Read the model definition and answer for the solid it produces. Units are mm, in the model's axes. A direction names the side the tool comes from. Coordinates: 2 decimals unless noted, no trailing zeros. Write each loop counter-clockwise with the first axis right and the second up, starting at its lowest first coordinate (ties: lowest second). Pieces come first, ordered by that corner, then holes. Notation, with made-up numbers: (-24, 10.25) -> (-12, 10.25) arc R31 ccw to (-12, 37.25) -> close; hole circle Ø2 at (24, 89). An arc over 180 degrees is marked (long way). Return JSON: item names as keys, results as strings.
from build123d import *

# Parameters (mm, degrees)
SKETCH_1_W           = 94
SKETCH_1_H           = 26
SKETCH_1_R           = 0.6
EXTRUDE_1_DEPTH      = 8
SKETCH_2_W           = 4.7
SKETCH_2_H           = 8.9
SKETCH_2_W_2         = 59.6
SKETCH_2_H_2         = 6.6
CUT_EXTRUDE_1_DEPTH  = 50.416596402
SKETCH_3_R           = 1.5
CUT_EXTRUDE_2_DEPTH  = 50.416596402
SKETCH_5_W           = 7.8
SKETCH_5_H           = 2.6
SKETCH_5_W_2         = 8.6
SKETCH_5_H_2         = 2
CUT_EXTRUDE_4_DEPTH  = 6
SKETCH_5_3_W         = 15.6
SKETCH_5_3_H         = 2
CUT_EXTRUDE_5_DEPTH  = 20
SKETCH_6_W           = 70
SKETCH_6_H           = 19.6
SKETCH_6_W_2         = 18.8
SKETCH_6_H_2         = 3
SKETCH_6_W_3         = 82.8
SKETCH_6_H_3         = 11
SKETCH_6_W_4         = 3.2
SKETCH_6_H_4         = 5.2
CUT_EXTRUDE_12_DEPTH = 2
SKETCH_7_W           = 6.7
SKETCH_7_H           = 7.7
CUT_EXTRUDE_13_DEPTH = 0.5
SKETCH_8_W           = 7.4
SKETCH_8_H           = 5.4
SKETCH_8_W_2         = 15.6
SKETCH_8_H_2         = 1.5
EXTRUDE_2_DEPTH      = 2.1
SKETCH_10_W          = 19.8
SKETCH_10_H          = 1.9
SKETCH_10_W_2        = 11.8
SKETCH_10_H_2        = 4.2
EXTRUDE_3_DEPTH      = 2
EXTRUDE_4_REACH      = 53.894
SKETCH_12_W          = 100
SKETCH_12_H          = 32.2
SKETCH_12_W_2        = 94
SKETCH_12_H_2        = 26.1
SKETCH_12_3_W        = 4.3
SKETCH_12_3_H        = 3
SKETCH_12_3_W_2      = 1
SKETCH_12_3_W_3      = 3.2
SKETCH_12_3_H_2      = 5.2
CUT_EXTRUDE_16_DEPTH = 54.133887492
SKETCH_13_W          = 94
SKETCH_13_H          = 0.1
EXTRUDE_5_DEPTH      = 8
SKETCH_14_W          = 1
SKETCH_14_H          = 8
CUT_EXTRUDE_17_DEPTH = 0.5
SKETCH_15_W          = 100
SKETCH_15_H          = 4
EXTRUDE_6_DEPTH      = 2
SKETCH_16_W          = 12
SKETCH_16_H          = 3.1
CUT_EXTRUDE_18_DEPTH = 55.479445665
SKETCH_17_R          = 1
CUT_EXTRUDE_19_DEPTH = 55.221859061
CUT_EXTRUDE_20_REACH = 104.313
SKETCH_18_W          = 8.9
SKETCH_18_H          = 4.7
SKETCH_19_W          = 4
SKETCH_19_H          = 1.5
CUT_EXTRUDE_21_DEPTH = 55.479445665


with BuildPart() as part:
    # 草图1 → 凸台-拉伸1 (new body)
    with BuildSketch(Plane(origin=(0, 0, 0), x_dir=(1, 0, 0), z_dir=(0, 1, 0))):
        Rectangle(SKETCH_1_W, SKETCH_1_H)
        with Locations(Location((-44, 10, 0), (0, 0, 270))):
            Circle(SKETCH_1_R, mode=Mode.SUBTRACT)
        with Locations(Location((-44, -10, 0), (0, 0, 270))):
            Circle(SKETCH_1_R, mode=Mode.SUBTRACT)
        with Locations(Location((44, 10, 0), (0, 0, 270))):
            Circle(SKETCH_1_R, mode=Mode.SUBTRACT)
        with Locations(Location((44, -10, 0), (0, 0, 270))):
            Circle(SKETCH_1_R, mode=Mode.SUBTRACT)
    extrude(amount=EXTRUDE_1_DEPTH)

    # 草图2 → 切除-拉伸1 (cut, through all)
    with BuildSketch(Plane.XZ):
        with Locations((-44.65, 2.65)):
            Rectangle(SKETCH_2_W, SKETCH_2_H)
        with Locations((-4.8, 0)):
            Rectangle(SKETCH_2_W_2, SKETCH_2_H_2)
    extrude(amount=-CUT_EXTRUDE_1_DEPTH, mode=Mode.SUBTRACT)

    # 草图3 → 切除-拉伸2 (cut, through all)
    with BuildSketch(Plane(origin=(0, 0, 0), x_dir=(-1, 0, 0), z_dir=(0, -1, 0))):
        with Locations(Location((27.5, -10, 0), (0, 0, 90))):
            Circle(SKETCH_3_R)
    extrude(amount=-CUT_EXTRUDE_2_DEPTH, mode=Mode.SUBTRACT)

    # 草图5 → 切除-拉伸4 (cut)
    with BuildSketch(Plane.XY.offset(13)):
        with Locations((-37.2, 6.7)):
            Rectangle(SKETCH_5_W, SKETCH_5_H)
        with Locations((-27.5, 7)):
            Rectangle(SKETCH_5_W_2, SKETCH_5_H_2)
    extrude(amount=-CUT_EXTRUDE_4_DEPTH, mode=Mode.SUBTRACT)

    # 草图5<3> → 切除-拉伸5 (cut)
    with BuildSketch(Plane.XY.offset(13)):
        with Locations((32.9, 7)):
            Rectangle(SKETCH_5_3_W, SKETCH_5_3_H)
    extrude(amount=-CUT_EXTRUDE_5_DEPTH, mode=Mode.SUBTRACT)

    # 草图6 → 切除-拉伸12 (cut)
    with BuildSketch(Plane(origin=(0, 8, 0), x_dir=(1, 0, 0), z_dir=(0, 1, 0))):
        with Locations((-7.8, 2.7)):
            Rectangle(SKETCH_6_W, SKETCH_6_H)
        with Locations((36.6, 0)):
            Rectangle(SKETCH_6_W_2, SKETCH_6_H_2)
        with Locations((0.3, -7)):
            Rectangle(SKETCH_6_W_3, SKETCH_6_H_3)
        with Locations((-44.4, 5.4)):
            Rectangle(SKETCH_6_W_4, SKETCH_6_H_4)
    extrude(amount=-CUT_EXTRUDE_12_DEPTH, mode=Mode.SUBTRACT)

    # 草图7 → 切除-拉伸13 (cut)
    with BuildSketch(Plane(origin=(0, 6, 0), x_dir=(1, 0, 0), z_dir=(0, 1, 0))):
        with Locations((-27.35, 7.15)):
            Rectangle(SKETCH_7_W, SKETCH_7_H)
    extrude(amount=-CUT_EXTRUDE_13_DEPTH, mode=Mode.SUBTRACT)

    # 草图8 → 凸台-拉伸2 (add)
    with BuildSketch(Plane.XY.offset(13)):
        with Locations((-37.2, 2.7)):
            Rectangle(SKETCH_8_W, SKETCH_8_H)
        with Locations((32.9, 0.75)):
            Rectangle(SKETCH_8_W_2, SKETCH_8_H_2)
    extrude(amount=EXTRUDE_2_DEPTH)

    # 草图10 → 凸台-拉伸3 (add)
    with BuildSketch(Plane.ZY.offset(47)):
        with Locations((0, 0.95)):
            Rectangle(SKETCH_10_W, SKETCH_10_H)
        with Locations((0, 2.1)):
            Rectangle(SKETCH_10_W_2, SKETCH_10_H_2)
    extrude(amount=EXTRUDE_3_DEPTH)

    # 凸台-拉伸4: up to this face of the body (flat: up to its plane)
    extrude_4_end = Plane(part.part.faces().sort_by_distance((-45.999719539, 0, 11.45))[0])
    # 草图12 → 凸台-拉伸4 (add, up to the picked face)
    with BuildSketch(Plane(origin=(0, 8, 0), x_dir=(1, 0, 0), z_dir=(0, 1, 0)), mode=Mode.PRIVATE) as extrude_4_sk1:
        Rectangle(SKETCH_12_W, SKETCH_12_H)
        with Locations((0, -0.05)):
            Rectangle(SKETCH_12_W_2, SKETCH_12_H_2, mode=Mode.SUBTRACT)
    extrude_4_tool1 = split(extrude(extrude_4_sk1.sketch, amount=-EXTRUDE_4_REACH, mode=Mode.PRIVATE), bisect_by=extrude_4_end, keep=Keep.BOTH, mode=Mode.PRIVATE)
    add(extrude_4_tool1.solids().sort_by(Axis((48.949436, 8, 0), (0, -1, 0)))[0])

    # 草图12<3> → 切除-拉伸16 (cut, through all)
    with BuildSketch(Plane(origin=(0, 8, 0), x_dir=(1, 0, 0), z_dir=(0, 1, 0))):
        Polygon((41.7, 13), (-42.8, 13), (-42.8, 12.5), (27.2, 12.5), (27.2, 7), (40.7, 7), (40.7, 1.5), (41.7, 1.5), align=None)
        Polygon((27.2, 12.5), (-42.8, 12.5), (-42.8, 8), (-42.8, 2.8), (-42.8, 1.8), (-42.8, -13.1), (41.7, -13.1), (41.7, -13), (40.7, -13), (40.7, -12.5), (41.7, -12.5), (41.7, -1.5), (41.7, 1.5), (40.7, 1.5), (40.7, 7), (27.2, 7), align=None)
        with Locations((43.85, 0)):
            Rectangle(SKETCH_12_3_W, SKETCH_12_3_H)
        with Locations((46.5, 0)):
            Rectangle(SKETCH_12_3_W_2, SKETCH_12_3_H)
        with Locations((-44.4, 5.4)):
            Rectangle(SKETCH_12_3_W_3, SKETCH_12_3_H_2)
        with Locations((-46.5, 5.4)):
            Rectangle(SKETCH_12_3_W_2, SKETCH_12_3_H_2)
        Polygon((-46, 2.8), (-47, 2.8), (-47, 1.8), (-42.8, 1.8), (-42.8, 2.8), align=None)
    extrude(amount=-CUT_EXTRUDE_16_DEPTH, mode=Mode.SUBTRACT)

    # 草图13 → 凸台-拉伸5 (add)
    with BuildSketch(Plane(origin=(0, 8, 0), x_dir=(1, 0, 0), z_dir=(0, 1, 0))):
        with Locations((0, -13.05)):
            Rectangle(SKETCH_13_W, SKETCH_13_H)
    extrude(amount=-EXTRUDE_5_DEPTH)

    # 草图14 → 切除-拉伸17 (cut)
    with BuildSketch(Plane(origin=(0, 0, 13), x_dir=(-1, 0, 0), z_dir=(0, 0, -1))):
        with Locations((-41.2, 4)):
            Rectangle(SKETCH_14_W, SKETCH_14_H)
    extrude(amount=CUT_EXTRUDE_17_DEPTH, mode=Mode.SUBTRACT)

    # 草图15 → 凸台-拉伸6 (add)
    with BuildSketch(Plane.XZ):
        with Locations((0, 18.1)):
            Rectangle(SKETCH_15_W, SKETCH_15_H)
        with Locations((0, -18.1)):
            Rectangle(SKETCH_15_W, SKETCH_15_H)
    extrude(amount=-EXTRUDE_6_DEPTH)

    # 草图16 → 切除-拉伸18 (cut, through all)
    with BuildSketch(Plane(origin=(0, 8, 0), x_dir=(1, 0, 0), z_dir=(0, 1, 0))):
        with Locations((-37.2, -14.55)):
            Rectangle(SKETCH_16_W, SKETCH_16_H)
    extrude(amount=-CUT_EXTRUDE_18_DEPTH, mode=Mode.SUBTRACT)

    # 草图17 → 切除-拉伸19 (cut, through all)
    with BuildSketch(Plane(origin=(0, 2, 0), x_dir=(1, 0, 0), z_dir=(0, 1, 0))):
        with Locations(Location((30, 18.1, 0), (0, 0, 270))):
            Circle(SKETCH_17_R)
        with Locations(Location((30, -18.1, 0), (0, 0, 270))):
            Circle(SKETCH_17_R)
        with Locations(Location((-30, 18.1, 0), (0, 0, 270))):
            Circle(SKETCH_17_R)
        with Locations(Location((-30, -18.1, 0), (0, 0, 270))):
            Circle(SKETCH_17_R)
    extrude(amount=-CUT_EXTRUDE_19_DEPTH, mode=Mode.SUBTRACT)

    # 切除-拉伸20: up to this face of the body (flat: up to its plane)
    cut_extrude_20_end = Plane(part.part.faces().sort_by_distance((41.7, 4, 7.25))[0])
    # 草图18 → 切除-拉伸20 (cut, up to the picked face)
    with BuildSketch(Plane(origin=(50, 0, 0), x_dir=(0, 0, -1), z_dir=(1, 0, 0)), mode=Mode.PRIVATE) as cut_extrude_20_sk1:
        with Locations((0, 2.35)):
            Rectangle(SKETCH_18_W, SKETCH_18_H)
    cut_extrude_20_tool1 = split(extrude(cut_extrude_20_sk1.sketch, amount=-CUT_EXTRUDE_20_REACH, mode=Mode.PRIVATE), bisect_by=cut_extrude_20_end, keep=Keep.BOTH, mode=Mode.PRIVATE)
    add(cut_extrude_20_tool1.solids().sort_by(Axis((50, 2.35, 0), (-1, 0, 0)))[0], mode=Mode.SUBTRACT)

    # 草图19 → 切除-拉伸21 (cut, through all)
    with BuildSketch(Plane(origin=(0, 8, 0), x_dir=(1, 0, 0), z_dir=(0, 1, 0))):
        with Locations((39.7, 13.75)):
            Rectangle(SKETCH_19_W, SKETCH_19_H)
    extrude(amount=-CUT_EXTRUDE_21_DEPTH, mode=Mode.SUBTRACT)


solid = part.part
1. A tool of negligible diameter and unlimited length cuts with its end or side. For faces 5 (the face through (46, 2, 4.45)), 6 (the face through (-47, 5, 16.1)), 7 (the face through (-1, 2, -18)), 8 (the face through (44, 6, 1.5)), from which of +Z, -Z, +X, -X, +Y, -Y can it reach the whole face along a straight path? Write none if from no direction.
Taken from the geometry:
{"face 5": "+X, -Y", "face 6": "+Z, +X, -X, +Y", "face 7": "-Z, +X, -X, +Y", "face 8": "+Y, -Y"}
2. The part is cut by section C-C (y = 6.5). Determine the outline of the cut face in (x, z).
Taken from the geometry:
{"outline": "(-50, -16.1) -> (50, -16.1) -> (50, 16.1) -> (-31.2, 16.1) -> (-31.2, 13) -> (41.7, 13) -> (41.7, 1.5) -> (47, 1.5) -> (47, -1.5) -> (41.7, -1.5) -> (41.7, -14.5) -> (37.7, -14.5) -> (37.7, -13) -> (-42.8, -13) -> (-42.8, -8) -> (-47, -8) -> (-47, 7.1) -> (-42.8, 7.1) -> (-42.8, 13) -> (-43.2, 13) -> (-43.2, 16.1) -> (-50, 16.1) -> close; hole circle Ø1.2 at (-44, -10); hole circle Ø1.2 at (-44, 10); hole circle Ø1.2 at (44, -10); hole circle Ø1.2 at (44, 10)"}
3. The part is cut by section A-A (z = 15). Determine the outline of the cut face in (x, y), then the cut area to 3 significant figures.
Taken from the geometry:
{"outline": "(-50, 0) -> (-43.2, 0) -> (-43.2, 8) -> (-50, 8) -> close; (-31.2, 0) -> (50, 0) -> (50, 8) -> (-31.2, 8) -> close", "area": "704 mm2"}
4. Flat-ended cylindrical pins translate along their axes: pin 1 Ø2 at (x, y) = (-44.5, 3.5) entering from -Z; pin 2 Ø1 at (x, y) = (43.5, 7) entering from +Z; pin 3 Ø0.7 at (x, z) = (-44, -10) entering from -Y; pin 4 Ø2.5 at (y, z) = (2, 1.5) entering from +X. Find the tip coordinate at first contact, or state that the pin passes through.
Taken from the geometry:
{"pin 1": "stops at z = -16.1", "pin 2": "stops at z = 16.1", "pin 3": "passes through", "pin 4": "stops at x = -47"}
5. The part is cut by section D-D (z = -3.5). Determine the outline of the cut face in (x, y), then the cut area to 3 significant figures.
Taken from the geometry:
{"outline": "(-50, 0) -> (-47, 0) -> (-47, 8) -> (-50, 8) -> close; (41.7, 4.7) -> (50, 4.7) -> (50, 8) -> (41.7, 8) -> close", "area": "51.4 mm2"}
6. For a pull along Z with two mould halves and no side action, classify faces 1 (the face through (-1, 1, 20.1)), 2 (the face through (-1, 2, 18)), 3 (the face through (-43.2, 4, 15)), 4 (the face through (-1, 5, -16.1)) as +Z half, -Z half, draft (parallel to the pull), parting line (faces both ways), or undercut.
Taken from the geometry:
{"face 1": "+Z half", "face 2": "draft", "face 3": "undercut", "face 4": "-Z half"}
7. The part is cut by section B-B (x = -11.5). Determine the outline of the cut face in (y, z).
Taken from the geometry:
{"outline": "(0, -20.1) -> (2, -20.1) -> (2, -16.1) -> (8, -16.1) -> (8, -13) -> (0, -13) -> close; (0, 13) -> (8, 13) -> (8, 16.1) -> (2, 16.1) -> (2, 20.1) -> (0, 20.1) -> close"}
8. Consider L1, parallel to Z at x = -44, y = 4; L2, parallel to X at y = 5.25, z = -10; L3, parallel to X at y = 0.9, z = -18.1. Determine where each line is inside the solid, lowest interval first.
Taken from the geometry:
{"L1": "z = -16.1 to -10.6, -9.4 to -8, 7.1 to 9.4, 10.6 to 16.1", "L2": "x = -50 to -44.6, -43.4 to -42.8, 41.7 to 43.4, 44.6 to 50", "L3": "x = -50 to -31, -29 to 29, 31 to 50"}
